from build123d import *
from OCP.BRepFilletAPI import BRepFilletAPI_MakeChamfer

# Parameters (mm, degrees)
SKETCH1_R           = 2.25
BOSS_EXTRUDE1_DEPTH = 3
CHAMFER2_SIZE       = 1
CHAMFER2_SIZE2      = 1.732050808
SKETCH2_R           = 2.25
CUT_EXTRUDE1_DEPTH  = 192.083751272
CHAMFER1_SIZE       = 3
CHAMFER3_SIZE       = 1
CHAMFER3_SIZE2      = 1.732050808


with BuildPart() as part:
    # Sketch1 → Boss-Extrude1 (new body)
    with BuildSketch(Plane(origin=(0, 0, 0), x_dir=(1, 0, 0), z_dir=(0, 1, 0))):
        with BuildLine():
            Line((-115, 0), (-156, 0))
            ThreePointArc((-156, 0), (-144.125207072, -59.698615449), (-110.308657865, -110.308657865))
            Line((-110.308657865, -110.308657865), (-81.317279836, -81.317279836))
            ThreePointArc((-81.317279836, -81.317279836), (-106.246146239, -44.008594722), (-115, 0))
        make_face()
        with Locations(Location((-149.708174067, -19.709455025, 0), (0, 0, 270))):
            Circle(SKETCH1_R, mode=Mode.SUBTRACT)
        with Locations(Location((-119.796354384, -91.92297578, 0), (0, 0, 270))):
            Circle(SKETCH1_R, mode=Mode.SUBTRACT)
    extrude(amount=BOSS_EXTRUDE1_DEPTH)

    # Chamfer2: one chamfer whose edges measure the first distance from different faces: ONE call of the kernel's chamfer builder (chamfer() names one face for all edges)
    chamfer2_edges_1 = [part.edges().sort_by_distance(p)[0] for p in [
        (-149.708174067, 3, 17.459455025),
    ]]
    chamfer2_side_1 = [part.faces().sort_by_distance(p)[0] for p in [
        (-149.708174067, 1.5, 17.459455025),
    ]]
    chamfer2_edges_2 = [part.edges().sort_by_distance(p)[0] for p in [
        (-119.796354384, 3, 89.67297578),
    ]]
    chamfer2_side_2 = [part.faces().sort_by_distance(p)[0] for p in [
        (-119.796354384, 1.5, 89.67297578),
    ]]
    chamfer2 = BRepFilletAPI_MakeChamfer(part.part.solid().wrapped)
    for e in chamfer2_edges_1:
        chamfer2.Add(CHAMFER2_SIZE, CHAMFER2_SIZE2, e.wrapped, chamfer2_side_1[0].wrapped)  # the first distance lies on this face
    for e in chamfer2_edges_2:
        chamfer2.Add(CHAMFER2_SIZE, CHAMFER2_SIZE2, e.wrapped, chamfer2_side_2[0].wrapped)  # the first distance lies on this face
    add(Compound.cast(chamfer2.Shape()), mode=Mode.REPLACE)

    # Sketch2 → Cut-Extrude1 (cut, through all)
    with BuildSketch(Plane(origin=(0, 3, 0), x_dir=(1, 0, 0), z_dir=(0, 1, 0))):
        with Locations(Location((-114.099122265, -47.261403897, 0), (0, 0, 270))):
            Circle(SKETCH2_R)
    extrude(amount=-CUT_EXTRUDE1_DEPTH, mode=Mode.SUBTRACT)

    # Chamfer1
    # the kernel refuses this chamfer: 3 mm, written as the material it takes off along each edge
    with BuildSketch(Plane(origin=(0, 3, 0), x_dir=(-0.9987770833709343, 0, -0.04944024406341062), z_dir=(0.04944024406341062, 0, -0.9987770833709343))) as chamfer1_piece_1:
        Polygon((156 - CHAMFER1_SIZE, 0), (156, -CHAMFER1_SIZE), (156, 0), align=None)
    revolve(axis=Axis((0, 3, 0), (0, 1, 0)), revolution_arc=50.667745228, mode=Mode.SUBTRACT)

    # Chamfer3
    chamfer3_edges = [part.edges().sort_by_distance(p)[0] for p in [
        (-114.099122265, 3, 45.011403897),
    ]]
    chamfer3_side = [part.faces().sort_by_distance(p)[0] for p in [
        (-114.099122265, 1.5, 45.011403897),
    ]]
    chamfer(chamfer3_edges, length=CHAMFER3_SIZE, length2=CHAMFER3_SIZE2, reference=chamfer3_side[0])


solid = part.part
Geometry check sheet. Reference: the model listing, model coordinates, mm. Round coordinates to 2 decimals unless told otherwise and drop trailing zeros. Order: outer loops, then holes, each group sorted by start corner. A loop starts at its lowest first (then second) coordinate and runs counter-clockwise, first axis right, second up. Notation, with made-up numbers: M -10.5,29 L 14.5,29 A16 ccw 14.5,49 Z; hole C 75,3 d8. An arc over 180 degrees is marked long. Answer in a Markdown table with one row per item.
(1) Go/stop test with flat-tipped pins: P1, Ø2.5, axis at x = -119.8, z = 91.92, coming from the -Y side; P2, Ø1, axis at x = -118.5, y = 1.5, coming from the +Z side; P3, Ø6, axis at x = -114.1, z = 47.26, coming from the +Y side; P4, Ø7, axis at x = -149.71, z = 19.71, coming from the +Y side. Record where each tip stops, or that it passes through.
Responses:
| item | result |
|---|---|
| P1 | passes through |
| P2 | stops at z = 100.11 |
| P3 | stops at y = 2.43 |
| P4 | stops at y = 2.72 |
(2) Sectioned sample at B-B, the plane x = -93. Record the cut outline in (y, z), and give its area (3 significant figures).
Responses:
| item | result |
|---|---|
| outline | M 0,67.65 L 3,67.65 L 3,93 L 0,93 Z |
| area | 76.1 mm² |
(3) Scan lines: probe 1 along X at (y, z) = (0.2, 49); probe 2 along Z at (x, y) = (-121, 1.4); probe 3 along X at (y, z) = (2, 90.5). Record each from-to range of solid material in increasing order. Write a range as from..to.
Responses:
| item | result |
|---|---|
| probe 1 | x = -147.89..-115.53, -112.67..-104.04 |
| probe 2 | z = 0..90.02, 93.82..96.23 |
| probe 3 | x = -124.6..-121.54, -118.05..-90.5 |
(4) Sectioned sample at A-A, the plane y = 1. Record the cut outline in (x, z).
Responses:
| item | result |
|---|---|
| outline | M -155,0 L -115,0 A115 cw -81.32,81.32 L -109.6,109.6 A155 ccw Z; hole C -149.71,19.71 d4.5; hole C -119.8,91.92 d4.5; hole C -114.1,47.26 d4.5 |
(5) Draft check along X on faces 1 (the face through (-141.85, 2.81, 57.84)), 2 (the face through (-111.87, 1.01, 46.97)), 3 (the face through (-106, 1.5, 44.6)), 4 (the face through (-118, 3, 53)). Enter one of: released by +X, released by -X, zero draft, split by the parting line, or undercut.
Responses:
| item | result |
|---|---|
| face 1 | released by -X |
| face 2 | undercut |
| face 3 | released by +X |
| face 4 | zero draft |
